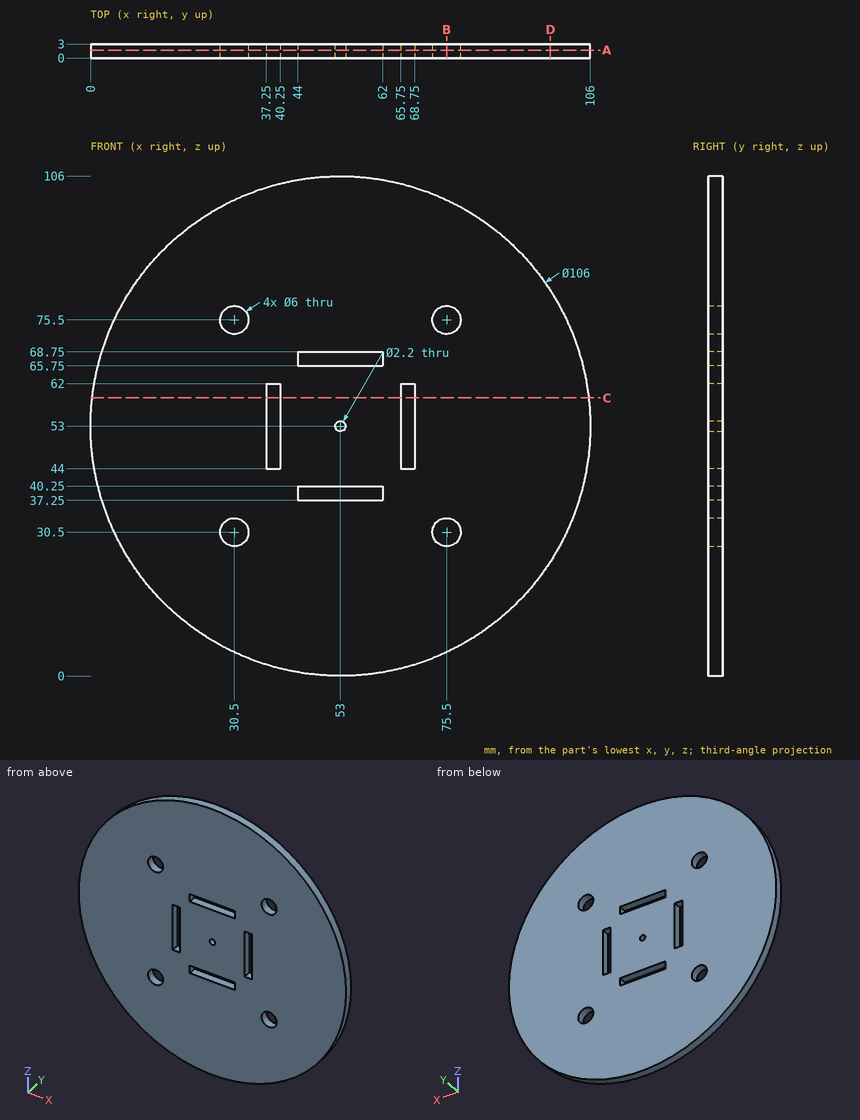
Design review of the part shown in the three views and the two pictorial views. Dimensions are in mm from the part's minimum x, y and z. Coordinates: 2 decimals unless noted, no trailing zeros. Loops run counter-clockwise (first coordinate to the right, second up) from the corner with the lowest first, then second, coordinate; pieces in that order, holes last. Notation, with made-up numbers: M 71,6.25 L 124,6.25 A28 cw 124,31.25 Z; hole C 64.25,67 d10. An arc over 180 degrees is marked long. One line per question, with ' | ' between items.
(1) For pin 1 Ø1.5 at (x, y) = (50.5, 1.5) entering from -Z; pin 2 Ø1.5 at (x, y) = (49.5, 1.5) entering from +Z; pin 3 Ø1 at (y, z) = (0.5, 49) entering from -X, all flat-tipped, find the tip position at first contact; note any pin that passes through.
Filled in:
pin 1: stops at z = 0.03 | pin 2: stops at z = 105.93 | pin 3: stops at x = 0.12
(2) Wall thickness on probe 1 along X at (y, z) = (1.95, 53); probe 2 along Z at (x, y) = (28, 1.15): over which ranges is each line inside the solid? List them lowest first.
Filled in:
probe 1: x = 0 to 37.25, 40.25 to 51.9, 54.1 to 65.75, 68.75 to 106 | probe 2: z = 6.27 to 28.84, 32.16 to 73.84, 77.16 to 99.73
(3) We need section A-A (y = 1.7). Count the separate pieces of the cut face and the enclosed holes in it, and give its area (3 significant figures).
Filled in:
separate pieces: 1 | enclosed holes: 9 | area: 8,490 mm^2
(4) We need section B-B (x = 75.5). Give the boundary of the cut face in (y, z).
Filled in:
outline: M 0,5.01 L 3,5.01 L 3,27.5 L 0,27.5 Z; M 0,33.5 L 3,33.5 L 3,72.5 L 0,72.5 Z; M 0,78.5 L 3,78.5 L 3,100.99 L 0,100.99 Z
(5) We need section D-D (x = 97.5). Give the boundary of the cut face in (y, z).
Filled in:
outline: M 0,24.21 L 3,24.21 L 3,81.79 L 0,81.79 Z
(6) We need section C-C (z = 59). Give the boundary of the cut face in (x, y).
Filled in:
outline: M 0.34,0 L 37.25,0 L 37.25,3 L 0.34,3 Z; M 40.25,0 L 65.75,0 L 65.75,3 L 40.25,3 Z; M 68.75,0 L 105.66,0 L 105.66,3 L 68.75,3 Z
